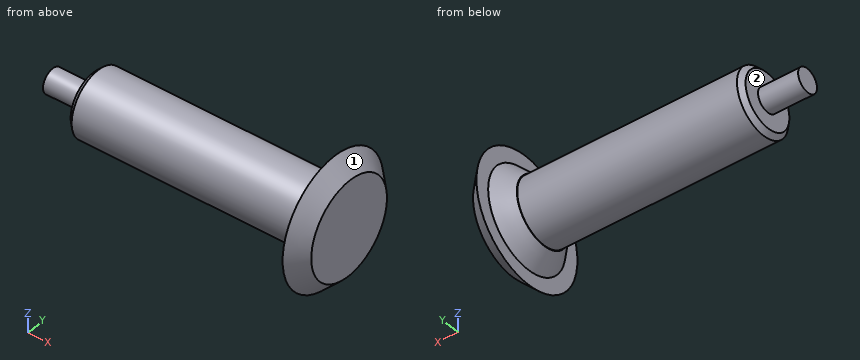
```python
from build123d import *

# Parameters (mm, degrees)
F0_W     = 25
F0_H     = 7.5
F2_SIZE2 = 3
F2_SIZE  = 3
F3_SIZE2 = 9.99999
F3_SIZE  = 9.99999
F4_SIZE2 = 9.99999
F4_SIZE  = 9.99999


# Not quite as in the source:
# - a fillet or chamfer is up to 0.001 mm smaller than in the source, because OpenCascade refuses the exact size


with BuildPart() as f1:
    # F0 (on Top) → F1 (revolve)
    with BuildSketch(Plane.XY):
        with Locations((-12.5, 3.75)):
            Rectangle(F0_W, F0_H)
        Polygon((0, 7.5), (0, 0), (140, 0), (140, 20.3452128917), (0, 20.3452128917), align=None)
        Polygon((140, 20.3452128917), (140, 0), (150, 0), (150, 30.6925382465), (140, 30.6925382465), align=None)
        Polygon((150, 30.6925382465), (150, 0), (160, 0), (160, 40), (150, 40), align=None)
    revolve(axis=Axis((70, 0, 0), (1, 0, 0)))

    # F2
    f2_edges = [f1.edges().sort_by_distance(p)[0] for p in [
        (0, -20.345213, 0),
    ]]
    chamfer(f2_edges, length=F2_SIZE, length2=F2_SIZE2)

    # F3 (size 10 and 10 in the source; OpenCascade refuses exactly that, so slightly less here)
    f3_edges = [f1.edges().sort_by_distance(p)[0] for p in [
        (140, -30.692538, 0),
    ]]
    chamfer(f3_edges, length=F3_SIZE, length2=F3_SIZE2)

    # F4 (size 10 and 10 in the source; OpenCascade refuses exactly that, so slightly less here)
    f4_edges = [f1.edges().sort_by_distance(p)[0] for p in [
        (160, -40, 0),
    ]]
    chamfer(f4_edges, length=F4_SIZE, length2=F4_SIZE2)


solid = f1.part
```
Verification items for the finished model (mm, model axes). Face numbers are marked on the shaded views. A direction names the side the tool comes from. Coordinates: 2 decimals unless noted, no trailing zeros. Write each loop counter-clockwise with the first axis right and the second up, starting at its lowest first coordinate (ties: lowest second). Pieces come first, ordered by that corner, then holes. Notation, with made-up numbers: M 40,63 L 52,63 A37 ccw 52,100 Z; hole C 30.25,57 d3. An arc over 180 degrees is marked long. One line per item, written item: value.
Item 1: Gauge pin test, flat ends, axial feed: pin 1 Ø8 at (x, y) = (128.5, -13.5) entering from +Z; pin 2 Ø10 at (y, z) = (-11, -22.5) entering from -X; pin 3 Ø10 at (x, z) = (71, -28.5) entering from +Y; pin 4 Ø8 at (x, z) = (104.5, -5.5) entering from +Y. Record the tip position at first contact, or that the pin passes through.
Check sheet entries:
pin 1: stops at z = 17.99
pin 2: stops at x = 2.7
pin 3: passes through
pin 4: stops at y = 20.29
Item 2: Section check D-D, the plane x = 147.5. Record the boundary of the cut face in (y, z).
Check sheet entries:
outline: C 0,0 d56.39
Item 3: Access from +Z, -Z, +X, -X, +Y, -Y to the whole of each face (thin tool, end or side, straight path). Record for the marked faces 1 and 2.
Check sheet entries:
face 1: +X
face 2: -X
Item 4: Scan lines: line 1 along Z through (x, y) = (69.5, 1); line 2 along X through (y, z) = (-12, -10.5); line 3 along X through (y, z) = (27, 13.5). Record each from-to range of solid material in increasing order.
Check sheet entries:
line 1: z = -20.32 to 20.32
line 2: x = 0 to 160
line 3: x = 149.49 to 159.81
Item 5: Section check C-C, the plane x = 91. Record the boundary of the cut face in (y, z), plus the area to 3 significant figures.
Check sheet entries:
outline: C 0,0 d40.69
area: 1,300 mm^2
